Print and shaded views of the part. All mm, measured from the part's lowest x, y and z. Coordinates: 2 decimals unless noted, no trailing zeros. Loops run counter-clockwise (first coordinate to the right, second up) from the corner with the lowest first, then second, coordinate; pieces in that order, holes last.
1) Saw through at D-D, the plane x = 7.75. Write the cut outline in (y, z) (1 decimal).
2) Wall check: line 1 along Y through (x, z) = (14, 0.65) (1 decimal); line 2 along Y through (x, z) = (7.75, 0.9) (1 decimal); line 3 along X through (y, z) = (19, 1.35) (1 decimal). Give the ranges that are in metal, low to high.
3) Saw through at A-A, the plane y = 16.5. Write the cut outline in (x, z) (1 decimal).
4) Pin check, flat tips, straight feed: pin 1 Ø2.5 at (x, y) = (3, 22.5) entering from +Z; pin 2 Ø5 at (x, y) = (15.5, 22) entering from -Z. Stop position of each tip, or through.
5) Saw through at C-C, the plane z = 1.35. Give the number of separate pieces and of enclosed holes in the cut face, and give its area (3 significant figures).
6) Saw through at B-B, the plane x = 14. Write the cut outline in (y, z) (1 decimal).
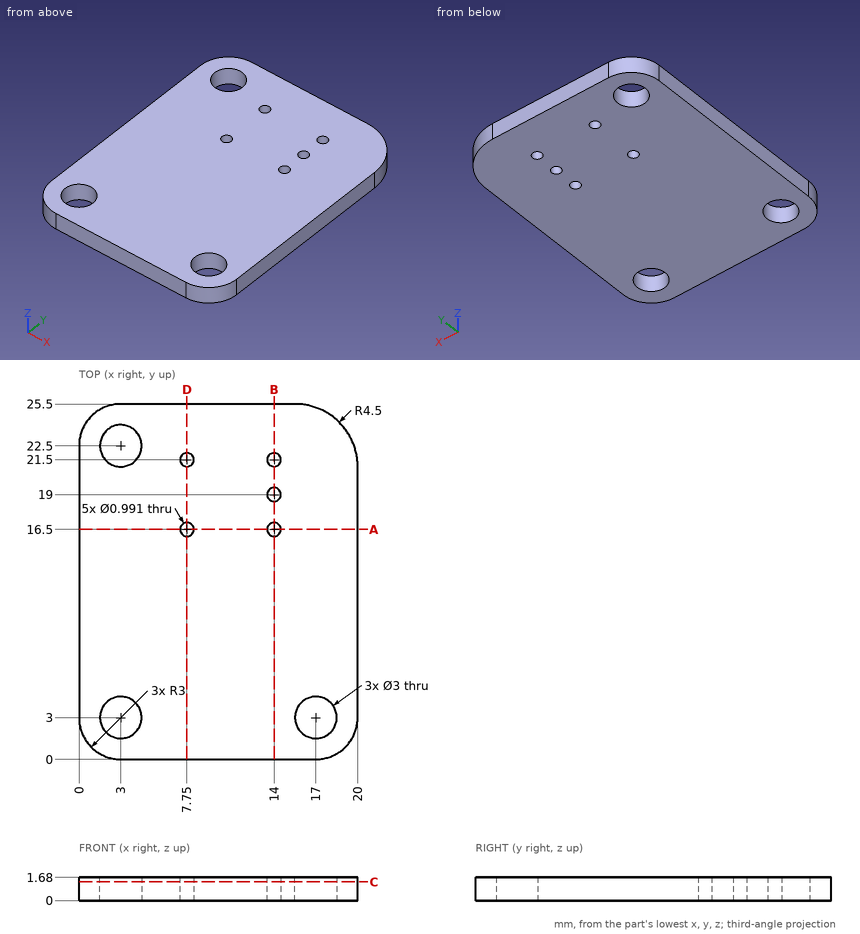
Data:
1. outline: (0, 0) - (16, 0) - (16, 1.7) - (0, 1.7) - close; (17, 0) - (21, 0) - (21, 1.7) - (17, 1.7) - close; (22, 0) - (25.5, 0) - (25.5, 1.7) - (22, 1.7) - close
2. line 1: y = 0 to 16, 17 to 18.5, 19.5 to 21, 22 to 25.5
2. line 2: y = 0 to 16, 17 to 21, 22 to 25.5
2. line 3: x = 0 to 13.5, 14.5 to 20
3. outline: (0, 0) - (7.3, 0) - (7.3, 1.7) - (0, 1.7) - close; (8.2, 0) - (13.5, 0) - (13.5, 1.7) - (8.2, 1.7) - close; (14.5, 0) - (20, 0) - (20, 1.7) - (14.5, 1.7) - close
4. pin 1: passes through
4. pin 2: stops at z = 0
5. separate pieces: 1
5. enclosed holes: 8
5. area: 475 mm2
6. outline: (0, 0) - (16, 0) - (16, 1.7) - (0, 1.7) - close; (17, 0) - (18.5, 0) - (18.5, 1.7) - (17, 1.7) - close; (19.5, 0) - (21, 0) - (21, 1.7) - (19.5, 1.7) - close; (22, 0) - (25.5, 0) - (25.5, 1.7) - (22, 1.7) - close
